Verification items for the finished model (mm, model axes). A direction names the side the tool comes from. Coordinates: 2 decimals unless noted, no trailing zeros. Loops run counter-clockwise (first coordinate to the right, second up) from the corner with the lowest first, then second, coordinate; pieces in that order, holes last.
Q1. Material ranges on probe 1 along Y at (x, z) = (0, 0.1); probe 2 along Y at (x, z) = (0, 3.3); probe 3 along Z at (x, y) = (-1.5, 1.5), recorded low to high.
Q2. Go/stop test with a flat-tipped pin: P1, Ø1.5, axis at x = 1.5, z = 2, coming from the -Y side. Record where the tip stops, or that it passes through.
Q3. Sectioned sample at C-C (z = 3.2). Enter the section's corners in (x, y).
Q4. Access from +Z, -Z, +X, -X, +Y, -Y to the whole of each face (thin tool, end or side, straight path). Record for faces 3 (the face through (-1.5, 0.07, 2.03)), 4 (the face through (2, -2, 3.7)).
Q5. Sectioned sample at A-A (y = 0). Enter the section's corners in (x, z), then the cut area to 3 significant figures.
Q6. Mould release check, pull along X, two halves, no side actions. Record for faces 1 (the face through (-0.867, -3.905, 1.972)), 2 (the face through (-2, -2, 0.3)): +X half, -X half, draft (parallel to the pull), parting line (faces both ways), or undercut.
Q7. Sectioned sample at D-D (y = 3). Enter the section's corners in (x, z), then the cut area to 3 significant figures.
```python
from build123d import *

# Parameters (mm, degrees)
SKETCH_1_R          = 4
EXTRUDE_1_DEPTH     = 4
SKETCH_2_R          = 1.5
CUT_EXTRUDE_1_DEPTH = 5
SKETCH_3_R          = 3.5
SKETCH_3_R_2        = 2
CUT_EXTRUDE_2_DEPTH = 0.3
SKETCH_4_R          = 3.5
SKETCH_4_R_2        = 2
CUT_EXTRUDE_3_DEPTH = 0.3


with BuildPart() as part:
    # 草圖1 → 填料-伸長1 (new body)
    with BuildSketch(Plane.XY):
        Circle(SKETCH_1_R)
    extrude(amount=EXTRUDE_1_DEPTH)

    # 草圖2 → 除料-伸長1 (cut, through all)
    with BuildSketch(Plane.XY.offset(4)):
        Circle(SKETCH_2_R)
    extrude(amount=-CUT_EXTRUDE_1_DEPTH, mode=Mode.SUBTRACT)

    # 草圖3 → 除料-伸長2 (cut)
    with BuildSketch(Plane.XY.offset(4)):
        Circle(SKETCH_3_R)
        Circle(SKETCH_3_R_2, mode=Mode.SUBTRACT)
    extrude(amount=-CUT_EXTRUDE_2_DEPTH, mode=Mode.SUBTRACT)

    # 草圖4 → 除料-伸長3 (cut)
    with BuildSketch(Plane(origin=(0, 0, 0), x_dir=(-1, 0, 0), z_dir=(0, 0, -1))):
        Circle(SKETCH_4_R)
        Circle(SKETCH_4_R_2, mode=Mode.SUBTRACT)
    extrude(amount=-CUT_EXTRUDE_3_DEPTH, mode=Mode.SUBTRACT)


solid = part.part
```
Geometry check:
1. probe 1: y = -4 to -3.5, -2 to -1.5, 1.5 to 2, 3.5 to 4
1. probe 2: y = -4 to -1.5, 1.5 to 4
1. probe 3: z = 0.3 to 3.7
2. P1: stops at y = -3.93
3. outline: circle Ø8 at (0, 0); hole circle Ø3 at (0, 0)
4. face 3: +Z, -Z
4. face 4: +Z
5. outline: (-4, 0) - (-3.5, 0) - (-3.5, 0.3) - (-2, 0.3) - (-2, 0) - (-1.5, 0) - (-1.5, 4) - (-2, 4) - (-2, 3.7) - (-3.5, 3.7) - (-3.5, 4) - (-4, 4) - close; (1.5, 0) - (2, 0) - (2, 0.3) - (3.5, 0.3) - (3.5, 0) - (4, 0) - (4, 4) - (3.5, 4) - (3.5, 3.7) - (2, 3.7) - (2, 4) - (1.5, 4) - close
5. area: 18.2 mm2
6. face 1: parting line
6. face 2: undercut
7. outline: (-2.65, 0) - (-1.8, 0) - (-1.8, 0.3) - (1.8, 0.3) - (1.8, 0) - (2.65, 0) - (2.65, 4) - (1.8, 4) - (1.8, 3.7) - (-1.8, 3.7) - (-1.8, 4) - (-2.65, 4) - close
7. area: 19.0 mm2
